Build history of the part. All positions in model axes, mm. Round coordinates to 2 decimals unless told otherwise and drop trailing zeros. Write each loop counter-clockwise with the first axis right and the second up, starting at its lowest first coordinate (ties: lowest second). Pieces come first, ordered by that corner, then holes. Notation, with made-up numbers: M 52.25,-10 L 86.25,-10 A24 cw 86.25,12 Z; hole C -19.75,-40 d4. An arc over 180 degrees is marked long. Use a Markdown table: item, result.
from build123d import *

# Parameters (mm, degrees)
F1_DEPTH = 10
F2_SIZE  = 4.99999
F4_D     = 5
F4_DEPTH = 20
F4_TIP   = 1.5021515476


# Not quite as in the source:
# - a fillet or chamfer is up to 0.001 mm smaller than in the source, because OpenCascade refuses the exact size


with BuildPart() as f1:
    # F0 (on Front) → F1 (new body)
    with BuildSketch(Plane.XZ):
        Polygon((0, 60.1269584066), (-15, 40.1269584066), (-15, -34.8730415934), (15, -34.8730415934), (15, 40.1269584066), align=None)
    extrude(amount=F1_DEPTH)

    # F2 (size 5 in the source; OpenCascade refuses exactly that, so slightly less here)
    f2_edges = [f1.edges().sort_by_distance(p)[0] for p in [
        (-15, -10, 2.626958),
        (-15, 0, 2.626958),
        (-7.5, -10, 50.126958),
        (-7.5, 0, 50.126958),
        (7.5, -10, 50.126958),
        (7.5, 0, 50.126958),
        (15, -10, 2.626958),
        (15, 0, 2.626958),
    ]]
    chamfer(f2_edges, length=F2_SIZE)

    # F4
    with Locations(Plane(origin=(0, 0, -34.8730415934), x_dir=(1, 0, 0), z_dir=(0, 0, -1))):
        with Locations((0, 5.1561156288)):
            Hole(F4_D / 2, depth=F4_DEPTH)
            with Locations((0, 0, -(F4_DEPTH + F4_TIP / 2))):  # 118° drill point
                Cone(0, F4_D / 2, F4_TIP, mode=Mode.SUBTRACT)


solid = f1.part
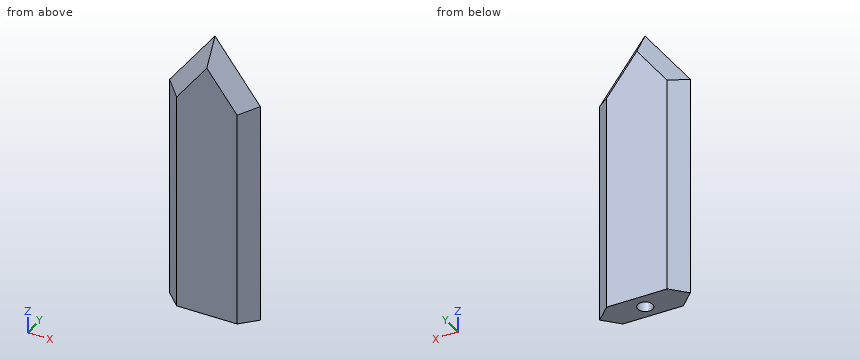
Q1. Cut at B-B on y = -9. Give the cut face in (x, z), and give its area (3 significant figures).
Response values:
| item | result |
|---|---|
| outline | M -11,-34.87 L 11,-34.87 L 11,38.79 L 0,53.46 L -11,38.79 Z |
| area | 1,780 mm2 |
Q2. Drill centre lines: L1, parallel to Y at x = 0, z = -27; L2, parallel to Y at x = -1, z = -21.5; L3, parallel to X at y = -5.75, z = -31. Where is each one in solid material? Low to high.
Response values:
| item | result |
|---|---|
| L1 | y = -10 to -7.66, -2.66 to 0 |
| L2 | y = -10 to -7.45, -2.86 to 0 |
| L3 | x = -14.25 to -2.43, 2.43 to 14.25 |
Q3. Drop flat-ended pins along their axis: P1, Ø6, axis at x = -4, y = -1.5, coming from the +Z side; P2, Ø1, axis at y = -7, z = 10, coming from the +X side; P3, Ø1, axis at y = -7.5, z = 44.5, coming from the -X side. Give the stop position or say it passes through.
Response values:
| item | result |
|---|---|
| P1 | stops at z = 55.36 |
| P2 | stops at x = 13.5 |
| P3 | stops at x = -9.32 |
